Check sheet for the modelled part. Datum: model origin and axes. Units: mm. A direction names the side the tool comes from. Round coordinates to 2 decimals unless told otherwise and drop trailing zeros. Write each loop counter-clockwise with the first axis right and the second up, starting at its lowest first coordinate (ties: lowest second). Pieces come first, ordered by that corner, then holes. Notation, with made-up numbers: (-3, 62) -> (38, 62) arc R20 ccw to (38, 86) -> close; hole circle Ø5 at (29, 62.25). An arc over 180 degrees is marked (long way). One line per item, written item: value.
from build123d import *

# Parameters (mm, degrees)
BOSS_EXTRUDE1_DEPTH = 4.5
SKETCH3_R           = 24.5
BOSS_EXTRUDE2_DEPTH = 33.45
CUT_EXTRUDE1_DEPTH  = 5


with BuildPart() as part:
    # Sketch1 → Boss-Extrude1 (new body)
    with BuildSketch(Plane(origin=(0, 0, 0), x_dir=(0, 1, 0), z_dir=(0, 0, 1))):
        Polygon((20.175580242, 11.933117582), (-0.246592851, 23.439123817), (-20.422173094, 11.506006235), (-20.175580242, -11.933117582), (0.246592851, -23.439123817), (20.422173094, -11.506006235), align=None)
    extrude(amount=BOSS_EXTRUDE1_DEPTH)

    # Sketch3 → Boss-Extrude2 (add)
    with BuildSketch(Plane.XY.offset(4.5)):
        Circle(SKETCH3_R)
    extrude(amount=BOSS_EXTRUDE2_DEPTH)

    # Sketch4 → Cut-Extrude1 (cut)
    with BuildSketch(Plane.XY.offset(37.95)):
        Polygon((11.506006235, 20.422173094), (-11.933117582, 20.175580242), (-23.439123817, -0.246592851), (-11.506006235, -20.422173094), (11.933117582, -20.175580242), (23.439123817, 0.246592851), align=None)
    extrude(amount=-CUT_EXTRUDE1_DEPTH, mode=Mode.SUBTRACT)


solid = part.part
Item 1: Depth check by flat-ended pin: pin 1 (10 mm diameter, centred on y = 14, z = 25.5, fed in from -X); pin 2 (3 mm diameter, centred on y = -6.5, z = 18.5, fed in from +X); pin 3 (8 mm diameter, centred on y = -9.5, z = 30, fed in from -X). Enter the tip coordinate at first touch or a pass-through.
Result set:
pin 1: x = -22.79
pin 2: x = 23.98
pin 3: x = -23.87
Item 2: Material ranges on line 1 along Z through (x, y) = (-7, 0.5); line 2 along Y through (x, z) = (9, 36); line 3 along Y through (x, z) = (21.5, 35), recorded low to high.
Result set:
line 1: 0 to 32.95
line 2: -22.79 to -20.21, 20.4 to 22.79
line 3: -11.75 to -3.2, 3.53 to 11.75
Item 3: Sectioned sample at C-C (z = 18). Enter the section's corners in (x, y), then the cut area to 3 significant figures.
Result set:
outline: circle Ø49 at (0, 0)
area: 1,890 mm^2
Item 4: Sectioned sample at A-A (y = -14). Enter the section's corners in (x, z).
Result set:
outline: (-20.11, 4.5) -> (-15.3, 4.5) -> (-15.3, 0) -> (15.41, 0) -> (15.41, 4.5) -> (20.11, 4.5) -> (20.11, 37.95) -> (15.41, 37.95) -> (15.41, 32.95) -> (-15.3, 32.95) -> (-15.3, 37.95) -> (-20.11, 37.95) -> close
Item 5: Sectioned sample at D-D (y = 21.5). Enter the section's corners in (x, z).
Result set:
outline: (-11.75, 4.5) -> (11.75, 4.5) -> (11.75, 37.95) -> (-11.75, 37.95) -> close
Item 6: Release check for a two-part mould opening along Y. For faces 1 (the flat face through (17.56, 10.19, 2.22)), 2 (the flat face through (0, 0, 32.95)), 3 (the cylindrical face through (13.17, 20.66, 20.99)) record: pulls with the +Y half, pulls with the -Y half, needs draft (parallel to the pull), parting line crosses it, or undercut.
Result set:
face 1: pulls with the +Y half
face 2: undercut
face 3: parting line crosses it
Item 7: Tool access check on faces 4 (the flat face through (17.606, -10.107, 35.485)), 5 (the flat face through (-17.606, 10.107, 2.218)), 6 (the flat face through (2, -22, 4.5)), 7 (the flat face through (17.606, -10.107, 2.218)), 8 (the flat face through (-17.56, -10.19, 2.22)). Record the directions out of +Z, -Z, +X, -X, +Y, -Y that give a thin tool (end or side, any length) a straight path to the whole face; none if there is none.
Result set:
face 4: +Z
face 5: -Z, -X, +Y
face 6: -Z
face 7: -Z, +X, -Y
face 8: -Z, -X, -Y
Item 8: Sectioned sample at B-B (x = -3.5). Enter the section's corners in (y, z), then the cut area to 3 significant figures.
Result set:
outline: (-24.25, 4.5) -> (-20.34, 4.5) -> (-20.34, 0) -> (20.26, 0) -> (20.26, 4.5) -> (24.25, 4.5) -> (24.25, 37.95) -> (20.26, 37.95) -> (20.26, 32.95) -> (-20.34, 32.95) -> (-20.34, 37.95) -> (-24.25, 37.95) -> close
area: 1,600 mm^2
